Source: CAD feature listing. Evaluate the final solid. Frame: model axes, mm. A direction names the side the tool comes from. Give positions to 0.01 mm unless a question says otherwise; leave off trailing zeros. Order: outer loops, then holes, each group sorted by start corner. A loop starts at its lowest first (then second) coordinate and runs counter-clockwise, first axis right, second up.
```python
from build123d import *

# Parameters (mm, degrees)
F1_DEPTH = 3.175
F3_DEPTH = 167.64


# Not quite as in the source:
# - a pattern or mirror of a feature is missing from the dataset's text; its kind, count and spacing are read off the source's solid


with BuildPart() as f1:
    # F0 (on Front) → F1 (new body, symmetric)
    with BuildSketch(Plane.XZ):
        with BuildLine():
            ThreePointArc((55.5949879174, -49.7616566718), (0, -74.6125), (-55.5949879174, -49.7616566718))
            Line((-55.5949879174, -49.7616566718), (-83.82, -49.7616566718))
            Line((-83.82, -49.7616566718), (-83.82, -81.5116566718))
            Line((-83.82, -81.5116566718), (83.82, -81.5116566718))
            Line((83.82, -81.5116566718), (83.82, -49.7616566718))
            Line((83.82, -49.7616566718), (55.5949879174, -49.7616566718))
        make_face()
    extrude(amount=F1_DEPTH, both=True)

    # F2 (on face) → F3 (join, through all)
    with BuildSketch(Plane.YZ.offset(83.82)):
        Polygon((-3.175, -81.5116566718), (-3.175, -75.1616566718), (-9.525, -80.7496566718), (-22.225, -80.7496566718), (-22.225, -81.5116566718), (-10.3909090909, -81.5116566718), align=None)
    f3 = extrude(amount=-F3_DEPTH)

    # F3_copies: F3 across plane
    add(f3.mirror(Plane.ZX))


solid = f1.part
```
1) Section query C-C, the plane z = -64. Return the cut outline in (x, y) (3 decimals), and give its area (3 significant figures).
Report:
outline: (-83.82, -3.175) - (-38.354, -3.175) - (-38.354, 3.175) - (-83.82, 3.175) - close; (38.354, -3.175) - (83.82, -3.175) - (83.82, 3.175) - (38.354, 3.175) - close
area: 577 mm2
2) Material intervals for L1, parallel to Y at x = -54, z = -56 (3 decimals); L2, parallel to Z at x = 11.5, y = 15.5; L3, parallel to X at y = 1, z = -61.5, sorted ascending.
Report:
L1: y = -3.175 to 3.175
L2: z = -81.51 to -80.75
L3: x = -83.82 to -42.25, 42.25 to 83.82
3) Section query D-D, the plane y = 18. Return the cut outline in (x, z).
Report:
outline: (-83.82, -81.51) - (83.82, -81.51) - (83.82, -80.75) - (-83.82, -80.75) - close
4) Section query A-A, the plane z = -72. Return the cut outline in (x, y) (3 decimals).
Report:
outline: (-83.82, -3.175) - (-19.571, -3.175) - (-19.571, 3.175) - (-83.82, 3.175) - close; (19.571, -3.175) - (83.82, -3.175) - (83.82, 3.175) - (19.571, 3.175) - close
5) Reachability of faces 1 (the flat face through (1, 16, -80.75)), 2 (the flat face through (-20, -3.175, -74)), 3 (the flat face through (70, 0, -49.762)) from +Z, -Z, +X, -X, +Y, -Y: full face, straight path, thin tool, end or side. Return the list, or none.
Report:
face 1: +Z, +X, -X, +Y
face 2: +Z, +X, -X, -Y
face 3: +Z, +X, -X, +Y, -Y
6) Pin query (flat end, axial travel): pin 1 (4 mm diameter, centred on x = -33, z = -65.5, fed in from +Y) (3 decimals); pin 2 (1.5 mm diameter, centred on x = -19.5, z = -72.5, fed in from -Y) (3 decimals); pin 3 (5 mm diameter, centred on y = -9.5, z = -76.5, fed in from +X); pin 4 (5 mm diameter, centred on x = 55.5, y = 14, fed in from +Z). Return the tip coordinate at first contact, or that it passes through.
Report:
pin 1: stops at y = 3.175
pin 2: stops at y = -3.175
pin 3: passes through
pin 4: stops at z = -80.75
7) Draft query along X for faces 4 (the flat face through (83.82, 0, -71)), 5 (the flat face through (-70, 0, -49.762)), 6 (the flat face through (-83.82, 0, -71)), 7 (the cylindrical face through (0.878, -0.044, -74.607)). Return one class per face: +X half, -X half, draft (parallel to the pull), parting line (faces both ways), or undercut.
Report:
face 4: +X half
face 5: draft
face 6: -X half
face 7: undercut
8) Section query B-B, the plane x = -43. Return the cut outline in (y, z) (3 decimals).
Report:
outline: (-22.225, -81.512) - (22.225, -81.512) - (22.225, -80.75) - (9.525, -80.75) - (3.175, -75.162) - (3.175, -60.976) - (-3.175, -60.976) - (-3.175, -75.162) - (-9.525, -80.75) - (-22.225, -80.75) - close
